For this review, take the finished solid that the model builds, in its own axes (mm). Face numbers are marked on the shaded views. A direction names the side the tool comes from. Coordinates: 2 decimals unless noted, no trailing zeros. Write each loop counter-clockwise with the first axis right and the second up, starting at its lowest first coordinate (ties: lowest second). Pieces come first, ordered by that corner, then holes. Notation, with made-up numbers: (52.5, -26.75) -> (108.5, -26.75) arc R35 cw to (108.5, 9.25) -> close; hole circle Ø6 at (-5, 88.25). An arc over 180 degrees is marked (long way). One line per item, written item: value. Start each with the question number.
1) Add section D-D (y = -3.5). State the section outline as (x, z) points, and give its area (3 significant figures).
2) Machinability: for the marked faces 3 and 4, which of the approach directions +Z, -Z, +X, -X, +Y, -Y give a long, thin tool a straight path to every point of the face, cutting with its end or side? Answer none if there is none.
3) Mouldability with a two-part tool opening along X and no side actions: class the marked faces 1 and 2 as released by +X, released by -X, zero draft, split by the parting line, or undercut.
4) For pin 1 Ø2 at (y, z) = (5, 4.5) entering from -X; pin 2 Ø6 at (x, z) = (-11, 7.5) entering from +Y; pin 3 Ø1 at (y, z) = (2, 9) entering from -X; pin 4 Ø3 at (x, y) = (0, 0) entering from +Z, all flat-tipped, find the tip position at first contact; note any pin that passes through.
5) For probe 1 along Y at (x, z) = (0, 4.25); probe 2 along Y at (x, z) = (-7.5, 2.5); probe 3 along X at (y, z) = (5, 7.75), list the stretches that pass through material, from the lowest coordinate up. Write a range as from..to.
6) Add section A-A (x = 0). State the section outline as (y, z) points.
7) Add section B-B (y = -10). State the section outline as (x, z) points, and give its area (3 significant figures).
8) Add section C-C (z = 9.5). State how many separate pieces and enclosed holes the cut face has, and give its area (3 significant figures).
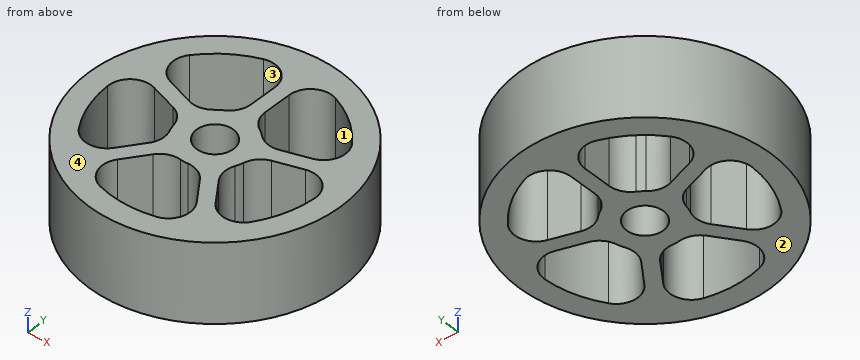
from build123d import *

# Parameters (mm, degrees)
F0_R     = 17.5
F0_R_2   = 2.55
F1_DEPTH = 11
F3_DEPTH = 25
F4_R     = 3


with BuildPart() as f1:
    # F0 (on Top) → F1 (new body)
    with BuildSketch(Plane.XY):
        Circle(F0_R)
        Circle(F0_R_2, mode=Mode.SUBTRACT)
    extrude(amount=F1_DEPTH)

    # F2 (on face) → F3 (cut)
    with BuildSketch(Plane.XY.offset(11)):
        with BuildLine():
            Line((-1, 4.898979), (-1, 14.465476))
            ThreePointArc((-1, 14.465476), (-8.522886, 11.730746), (-13.448468, 5.421134))
            Line((-13.448468, 5.421134), (-4.350189, 2.464924))
            ThreePointArc((-4.350189, 2.464924), (-2.938926, 4.045085), (-1, 4.898979))
        make_face()
        with BuildLine():
            Line((4.350189, 2.464924), (13.448468, 5.421134))
            ThreePointArc((13.448468, 5.421134), (8.522886, 11.730746), (1, 14.465476))
            Line((1, 14.465476), (1, 4.898979))
            ThreePointArc((1, 4.898979), (2.938926, 4.045085), (4.350189, 2.464924))
        make_face()
        with BuildLine():
            ThreePointArc((9.311611, -11.115031), (13.139033, -6.133174), (14.5, 0))
            ThreePointArc((14.5, 0), (14.391218, 1.772811), (14.066502, 3.519021))
            Line((14.066502, 3.519021), (4.968223, 0.562811))
            ThreePointArc((4.968223, 0.562811), (4.99205, 0.281854), (5, 0))
            ThreePointArc((5, 0), (4.660624, -1.810687), (3.688565, -3.375572))
            Line((3.688565, -3.375572), (9.311611, -11.115031))
        make_face()
        with BuildLine():
            ThreePointArc((-7.693577, -12.290601), (0, -14.5), (7.693577, -12.290601))
            Line((7.693577, -12.290601), (2.070531, -4.551143))
            ThreePointArc((2.070531, -4.551143), (0, -5), (-2.070531, -4.551143))
            Line((-2.070531, -4.551143), (-7.693577, -12.290601))
        make_face()
        with BuildLine():
            ThreePointArc((-14.066502, 3.519021), (-13.790319, -4.480746), (-9.311611, -11.115031))
            Line((-9.311611, -11.115031), (-3.688565, -3.375572))
            ThreePointArc((-3.688565, -3.375572), (-4.755283, -1.545085), (-4.968223, 0.562811))
            Line((-4.968223, 0.562811), (-14.066502, 3.519021))
        make_face()
    extrude(amount=-F3_DEPTH, mode=Mode.SUBTRACT)

    # F4
    f4_edges = [f1.edges().sort_by_distance(p)[0] for p in [
        (-1, 4.898979, 5.5),
        (-4.350189, 2.464924, 5.5),
        (1, 4.898979, 5.5),
        (4.350189, 2.464924, 5.5),
        (3.688565, -3.375572, 5.5),
        (4.968223, 0.562811, 5.5),
        (2.070531, -4.551143, 5.5),
        (-2.070531, -4.551143, 5.5),
        (-4.968223, 0.562811, 5.5),
        (-3.688565, -3.375572, 5.5),
        (13.448468, 5.421134, 5.5),
        (14.066502, 3.519021, 5.5),
        (1, 14.465476, 5.5),
        (-1, 14.465476, 5.5),
        (-13.448468, 5.421134, 5.5),
        (9.311611, -11.115031, 5.5),
        (-9.311611, -11.115031, 5.5),
        (-14.066502, 3.519021, 5.5),
        (7.693577, -12.290601, 5.5),
        (-7.693577, -12.290601, 5.5),
    ]]
    fillet(f4_edges, radius=F4_R)


solid = f1.part
Numbers:
1. outline: (-17.15, 0) -> (-14.07, 0) -> (-14.07, 11) -> (-17.15, 11) -> close; (-4.32, 0) -> (4.32, 0) -> (4.32, 11) -> (-4.32, 11) -> close; (14.07, 0) -> (17.15, 0) -> (17.15, 11) -> (14.07, 11) -> close
1. area: 163 mm²
2. face 3: +Z, -Z
2. face 4: +Z, +X, -X, +Y, -Y
3. face 1: undercut
3. face 2: zero draft
4. pin 1: x = -17.04
4. pin 2: y = 15.56
4. pin 3: x = -17.44
4. pin 4: through
5. probe 1: -17.5..-14.5, -5..-2.55, 2.55..17.5
5. probe 2: -15.81..-8.54, 1.39..3.49, 12.41..15.81
5. probe 3: -16.77..-11.12, -1.7..1.7, 11.12..16.77
6. outline: (-17.5, 0) -> (-14.5, 0) -> (-14.5, 11) -> (-17.5, 11) -> close; (-5, 0) -> (-2.55, 0) -> (-2.55, 11) -> (-5, 11) -> close; (2.55, 0) -> (17.5, 0) -> (17.5, 11) -> (2.55, 11) -> close
7. outline: (-14.36, 0) -> (-5.9, 0) -> (-5.9, 11) -> (-14.36, 11) -> close; (5.9, 0) -> (14.36, 0) -> (14.36, 11) -> (5.9, 11) -> close
7. area: 186 mm²
8. separate pieces: 1
8. enclosed holes: 6
8. area: 495 mm²
